Source: CAD feature listing. Evaluate the final solid. Frame: model axes, mm. Coordinates: 2 decimals unless noted, no trailing zeros. Order: outer loops, then holes, each group sorted by start corner. A loop starts at its lowest first (then second) coordinate and runs counter-clockwise, first axis right, second up. Notation, with made-up numbers: (-9, 81.5) - (22, 81.5) arc R26 ccw to (22, 100.5) - close; hole circle Ø4 at (-33.75, 2.25). An arc over 180 degrees is marked (long way). One line per question, with ' | ' between items. Start each with the question number.
(1) Contact query for a flat-ended pin moving along its axis: P1, Ø2, axis at x = 2.5, y = 3, coming from the -Z side. Output: stop coordinate, or through.
(2) Line query: line 1 along Y through (x, z) = (3.5, 0); line 2 along X through (y, z) = (4, -0.1); line 3 along Y through (x, z) = (4, -0.2). Output: solid intervals per line, ascending.
(3) Section C-C (y = 3). Return the cut outline in (x, z).
(4) Section B-B (x = 3.75). Return the cut outline in (y, z).
(5) Section A-A (z = 0). Return the cut outline in (x, y).
from build123d import *

# Parameters (mm, degrees)
SKETCH4_R = 0.3
FILLET1_R = 0.1


with BuildPart() as part:
    # Sweep1: sweep along a path in Sketch3
    with BuildLine(Plane.XY) as sweep1_path:
        Line((0, 0), (0, 5.5))
        ThreePointArc((0, 5.5), (0.292893219, 6.207106781), (1, 6.5))
        Line((1, 6.5), (6, 6.5))
    # Sketch4 → Sweep1 (sweep)
    with BuildSketch(Plane(origin=(0, 0, 0), x_dir=(1, 0, 0), z_dir=(0, 1, 0))):
        Circle(SKETCH4_R)
    sweep(path=sweep1_path.line)

    # Fillet1
    fillet1_edges = [part.edges().sort_by_distance(p)[0] for p in [
        (-0.3, 0, 0),
        (6, 6.8, 0),
    ]]
    fillet(fillet1_edges, radius=FILLET1_R)


solid = part.part
Response values:
1) P1: passes through
2) line 1: y = 6.2 to 6.8 | line 2: x = -0.28 to 0.28 | line 3: y = 6.28 to 6.72
3) outline: circle Ø0.6 at (0, 0)
4) outline: circle Ø0.6 at (6.5, 0)
5) outline: (-0.3, 0.1) arc R0.1 ccw to (-0.2, 0) - (0.2, 0) arc R0.1 ccw to (0.3, 0.1) - (0.3, 5.5) arc R0.7 cw to (1, 6.2) - (5.9, 6.2) arc R0.1 ccw to (6, 6.3) - (6, 6.7) arc R0.1 ccw to (5.9, 6.8) - (1, 6.8) arc R1.3 ccw to (-0.3, 5.5) - close
